Model file for the job. Use its own axes, mm. A direction names the side the tool comes from. Give positions to 0.01 mm unless a question says otherwise; leave off trailing zeros. Loops run counter-clockwise (first coordinate to the right, second up) from the corner with the lowest first, then second, coordinate; pieces in that order, holes last. Notation, with made-up numbers: M -32,-30 L 22,-30 A18 cw 22,-2 Z; hole C 82.25,1 d8. An arc over 180 degrees is marked long. Answer in a Markdown table with one row per item.
```python
from build123d import *

# Parameters (mm, degrees)
F0_R     = 63.5
F1_DEPTH = 76.2
F2_R     = 63.5
F2_R_2   = 38.354
F3_DEPTH = 50.8
F4_SIZE2 = 1.27
F4_SIZE  = 4.7397045256
F5_SIZE  = 5.08


with BuildPart() as f1:
    # F0 (on Front) → F1 (new body)
    with BuildSketch(Plane.XZ):
        Circle(F0_R)
    extrude(amount=F1_DEPTH)

    # F2 (on face) → F3 (cut)
    with BuildSketch(Plane.XZ.offset(76.2)):
        Circle(F2_R)
        Circle(F2_R_2, mode=Mode.SUBTRACT)
    extrude(amount=-F3_DEPTH, mode=Mode.SUBTRACT)

    # F4
    f4_edges = [f1.edges().sort_by_distance(p)[0] for p in [
        (-38.354, -76.2, 0),
    ]]
    f4_side = f1.faces().sort_by_distance((-38.354, -50.8, 0))[0]
    chamfer(f4_edges, length=F4_SIZE, length2=F4_SIZE2, reference=f4_side)

    # F5
    f5_edges = [f1.edges().sort_by_distance(p)[0] for p in [
        (-63.5, 0, 0),
    ]]
    chamfer(f5_edges, length=F5_SIZE)


solid = f1.part
```
(1) Which spindle directions (+Z, -Z, +X, -X, +Y, -Y) get a long thin tool onto all of the face, cutting with end or side? Do faces 1 (the flat face through (27.3, -25.4, -27.3)), 2 (the cylindrical face through (-13.77, -15.1, -61.99)). Say none if no direction does.
Established:
| item | result |
|---|---|
| face 1 | -Y |
| face 2 | +Y, -Y |
(2) Wall check: L1, parallel to Y at x = 11, z = -56; L2, parallel to X at y = -13, z = -1.5; L3, parallel to X at y = -67.5, z = 19.5. Give the ranges that are in metal, low to high.
Established:
| item | result |
|---|---|
| L1 | y = -25.4 to 0 |
| L2 | x = -63.48 to 63.48 |
| L3 | x = -33.03 to 33.03 |
(3) Flat gauge pins, fed straight in: P1, Ø10, axis at y = -15, z = -29.5, coming from the -X side; P2, Ø1, axis at x = 14, y = -48.5, coming from the -Z side; P3, Ø4, axis at y = -61, z = -16, coming from the -X side; P4, Ø10, axis at x = -37.5, z = 22, coming from the +Y side. Where does each tip first touch, or does it go through?
Established:
| item | result |
|---|---|
| P1 | stops at x = -58.58 |
| P2 | stops at z = -35.9 |
| P3 | stops at x = -35.71 |
| P4 | stops at y = 0 |
(4) Saw through at C-C, the plane y = -36.5. Give the cut face in (x, z).
Established:
| item | result |
|---|---|
| outline | C 0,0 d76.71 |
(5) Saw through at A-A, the plane x = 0. Give the cut face in (y, z), and give its area (3 significant figures).
Established:
| item | result |
|---|---|
| outline | M -76.2,-37.08 L -71.46,-38.35 L -25.4,-38.35 L -25.4,-63.5 L -5.08,-63.5 L 0,-58.42 L 0,58.42 L -5.08,63.5 L -25.4,63.5 L -25.4,38.35 L -71.46,38.35 L -76.2,37.08 Z |
| area | 7,090 mm2 |
(6) Saw through at B-B, the plane z = 0. Give the cut face in (x, y).
Established:
| item | result |
|---|---|
| outline | M -63.5,-25.4 L -38.35,-25.4 L -38.35,-71.46 L -37.08,-76.2 L 37.08,-76.2 L 38.35,-71.46 L 38.35,-25.4 L 63.5,-25.4 L 63.5,-5.08 L 58.42,0 L -58.42,0 L -63.5,-5.08 Z |
